from build123d import *

# Parameters (mm, degrees)
SKETCH_R      = 2.05
PAD_DEPTH     = 7
SKETCH001_R   = 5
SKETCH001_R_2 = 2.05
PAD001_DEPTH  = 20


with BuildPart() as part:
    # Sketch → Pad (new body)
    with BuildSketch(Plane.XY):
        with BuildLine():
            ThreePointArc((-4, 5), (-4.707107, 4.707107), (-5, 4))
            Line((-5, -4), (-5, 4))
            ThreePointArc((-5, -4), (-4.707107, -4.707107), (-4, -5))
            Line((29, -5), (-4, -5))
            ThreePointArc((29, -5), (29.707107, -4.707107), (30, -4))
            Line((30, 4), (30, -4))
            ThreePointArc((30, 4), (29.707107, 4.707107), (29, 5))
            Line((-4, 5), (29, 5))
        make_face()
        Circle(SKETCH_R, mode=Mode.SUBTRACT)
        with Locations((15, 0)):
            Circle(SKETCH_R, mode=Mode.SUBTRACT)
        with Locations((25, 0)):
            Circle(SKETCH_R, mode=Mode.SUBTRACT)
    extrude(amount=PAD_DEPTH)

    # Sketch001 → Pad001 (join)
    with BuildSketch(Plane.XY):
        Circle(SKETCH001_R)
        Circle(SKETCH001_R_2, mode=Mode.SUBTRACT)
    extrude(amount=PAD001_DEPTH)


solid = part.part
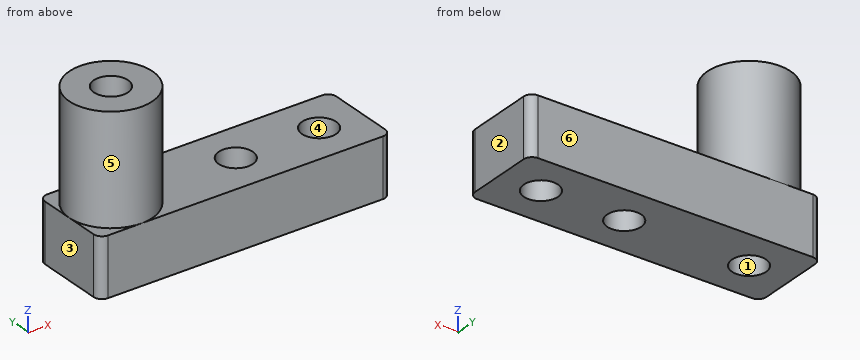
Geometry check sheet. Reference: the model listing, model coordinates, mm. Face numbers are marked on the shaded views. A direction names the side the tool comes from. Round coordinates to 2 decimals unless told otherwise and drop trailing zeros. Write each loop counter-clockwise with the first axis right and the second up, starting at its lowest first coordinate (ties: lowest second). Pieces come first, ordered by that corner, then holes.
Item 1: Access from +Z, -Z, +X, -X, +Y, -Y to the whole of each face (thin tool, end or side, straight path). Record for the marked faces 5 and 6.
Determined:
face 5: +Z
face 6: +Z, -Z, +X, -X, +Y
Item 2: Section check B-B (y = -0.5). Give the number of separate pieces and of enclosed holes in the cut face, plus the area to 3 significant figures.
Determined:
separate pieces: 4
enclosed holes: 0
area: 239 mm2
Item 3: Section check D-D (y = -2.5). Record the boundary of the cut face in (x, z), plus the area to 3 significant figures.
Determined:
outline: (-5, 0) - (30, 0) - (30, 7) - (4.33, 7) - (4.33, 20) - (-4.33, 20) - (-4.33, 7) - (-5, 7) - close
area: 358 mm2
Item 4: Mould release check, pull along X, two halves, no side actions. Record for the marked faces 1, 2, 3 and 4: +X half, -X half, draft (parallel to the pull), parting line (faces both ways), or undercut.
Determined:
face 1: undercut
face 2: +X half
face 3: -X half
face 4: undercut
Item 5: Material ranges on line 1 along Y through (x, z) = (15, 3); line 2 along Z through (x, y) = (10, 0.75); line 3 along X through (y, z) = (-3, 14.5), recorded low to high.
Determined:
line 1: y = -5 to -2.05, 2.05 to 5
line 2: z = 0 to 7
line 3: x = -4 to 4
Item 6: Go/stop test with flat-tipped pins: pin 1 Ø4.5 at (x, y) = (25, 0) entering from +Z; pin 2 Ø2.5 at (x, y) = (0, 0) entering from -Z; pin 3 Ø3 at (y, z) = (-2, 15.5) entering from +X. Record where each tip stops, or that it passes through.
Determined:
pin 1: stops at z = 7
pin 2: passes through
pin 3: stops at x = 4.97
Item 7: Section check A-A (x = 15). Record the boundary of the cut face in (y, z), plus the area to 3 significant figures.
Determined:
outline: (-5, 0) - (-2.05, 0) - (-2.05, 7) - (-5, 7) - close; (2.05, 0) - (5, 0) - (5, 7) - (2.05, 7) - close
area: 41.3 mm2
Item 8: Section check C-C (z = 11.25). Record the boundary of the cut face in (x, y).
Determined:
outline: circle Ø10 at (0, 0); hole circle Ø4.1 at (0, 0)
